Here's how the part is built. I have some questions about the finished solid (model axes, mm). Face numbers are marked on the shaded views. A direction names the side the tool comes from. Round coordinates to 2 decimals unless told otherwise and drop trailing zeros. Loops run counter-clockwise (first coordinate to the right, second up) from the corner with the lowest first, then second, coordinate; pieces in that order, holes last. Notation, with made-up numbers: (51, 50) -> (92, 50) arc R37 cw to (92, 86) -> close; hole circle Ø11 at (-23, 36). An arc over 180 degrees is marked (long way). One line per item, written item: value. Start each with the question number.
```python
from build123d import *

# Parameters (mm, degrees)
SKETCH2_W           = 18
SKETCH2_H           = 18
BOSS_EXTRUDE1_DEPTH = 4.3
BOSS_EXTRUDE2_DEPTH = 6.44
SHELL2_T            = -0.6
SKETCH5_R           = 4
CUT_EXTRUDE1_DEPTH  = 17.653756333


with BuildPart() as part:
    # Sketch2 → Boss-Extrude1 (new body)
    with BuildSketch(Plane(origin=(0, 0, 0), x_dir=(0, 0, -1), z_dir=(1, 0, 0))):
        Rectangle(SKETCH2_W, SKETCH2_H)
    extrude(amount=BOSS_EXTRUDE1_DEPTH)

    # Sketch4 → Boss-Extrude2 (add)
    with BuildSketch(Plane(origin=(4.3, 0, 0), x_dir=(0, 0, -1), z_dir=(1, 0, 0))):
        with BuildLine():
            Line((-2.8, -7.6), (2.8, -7.6))
            Line((2.8, -7.6), (2.8, -4))
            ThreePointArc((2.8, -4), (0, 7.306599665), (-2.8, -4))
            Line((-2.8, -4), (-2.8, -7.6))
        make_face()
    extrude(amount=BOSS_EXTRUDE2_DEPTH)

    # Shell2
    shell2_openings = [part.faces().sort_by_distance(p)[0] for p in [
        (0, 0, 0),
    ]]
    offset(amount=SHELL2_T, openings=shell2_openings, kind=Kind.INTERSECTION)

    # Sketch5 → Cut-Extrude1 (cut, through all)
    with BuildSketch(Plane(origin=(10.74, 0, 0), x_dir=(0, 0, -1), z_dir=(1, 0, 0))):
        with Locations((0, 1.306599665)):
            Circle(SKETCH5_R)
    extrude(amount=-CUT_EXTRUDE1_DEPTH, mode=Mode.SUBTRACT)


solid = part.part
```
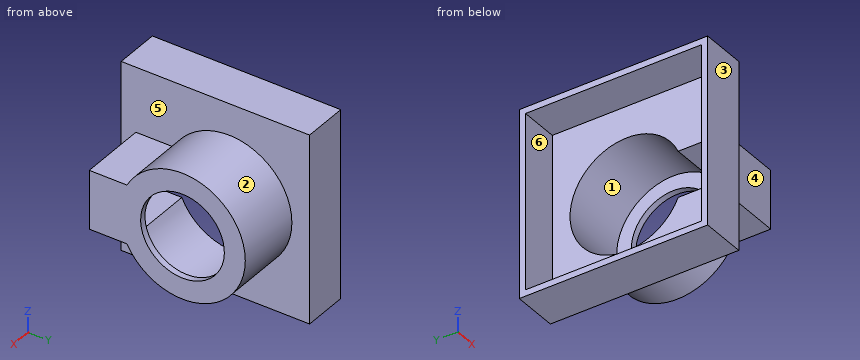
Q1. If I drill on line 1 along Z through (x, y) = (3.25, -4.5); line 2 along Y through (x, z) = (10.65, 0), over which ranges is the centre line in solid material (lowest first)?
Q2. If we mould it in two halves opening along Y, with no side actions, what happens to the marked faces 1, 2 and 3? For each: released by +Y, released by -Y, zero draft, split by the parting line, or undercut.
Q3. I want a section at A-A on z = 0. Please give me the cut outline in (x, y).
Q4. I want a section at C-C on y = -1. Please give me the cut outline in (x, z).
Q5. Will these pins go through, and if not, where does the flat tip stop? P1, Ø3, axis at y = -1.5, z = -1, coming from the -X side; P2, Ø2.5, axis at x = 8.5, y = -5.5, coming from the +Z side; P3, Ø2, axis at x = 8.5, z = 5, coming from the +Y side; P4, Ø2, axis at y = -1, z = 0, coming from the +X side.
Q6. Which directions (+Z, -Z, +X, -X, +Y, -Y) give clear straight access to the entire face, cutting with the end or side of a thin tool? Please do the marked faces 4, 5 and 6.
Q7. I want a section at B-B on x = 8.75. Please give me the cut outline in (y, z).
Q8. I want a section at D-D on x = 1. Please give me the cut outline in (y, z).
Answers below:
1. line 1: z = -9 to -8.4, 8.4 to 9
1. line 2: y = -7.6 to -2.69, 5.31 to 7.31
2. face 1: undercut
2. face 2: split by the parting line
2. face 3: released by -Y
3. outline: (0, -9) -> (4.3, -9) -> (4.3, -7.6) -> (10.74, -7.6) -> (10.74, -2.69) -> (10.14, -2.69) -> (10.14, -7) -> (3.7, -7) -> (3.7, -8.4) -> (0, -8.4) -> close; (0, 8.4) -> (3.7, 8.4) -> (3.7, 6.71) -> (10.14, 6.71) -> (10.14, 5.31) -> (10.74, 5.31) -> (10.74, 7.31) -> (4.3, 7.31) -> (4.3, 9) -> (0, 9) -> close
4. outline: (0, -9) -> (4.3, -9) -> (4.3, -5.54) -> (10.74, -5.54) -> (10.74, -3.27) -> (10.14, -3.27) -> (10.14, -4.88) -> (3.7, -4.88) -> (3.7, -8.4) -> (0, -8.4) -> close; (0, 8.4) -> (3.7, 8.4) -> (3.7, 4.88) -> (10.14, 4.88) -> (10.14, 3.27) -> (10.74, 3.27) -> (10.74, 5.54) -> (4.3, 5.54) -> (4.3, 9) -> (0, 9) -> close
5. P1: stops at x = 10.14
5. P2: stops at z = 2.8
5. P3: stops at y = 5.78
5. P4: passes through
6. face 4: +Z, -Z, +X, -Y
6. face 5: +X
6. face 6: -X
7. outline: (-7.6, -2.8) -> (-4, -2.8) arc R6 ccw (long way) to (-4, 2.8) -> (-7.6, 2.8) -> close; hole (-7, -2.2) -> (-3.62, -2.2) arc R5.4 ccw (long way) to (-3.62, 2.2) -> (-7, 2.2) -> close
8. outline: (-9, -9) -> (9, -9) -> (9, 9) -> (-9, 9) -> close; hole (-8.4, -8.4) -> (8.4, -8.4) -> (8.4, 8.4) -> (-8.4, 8.4) -> close
